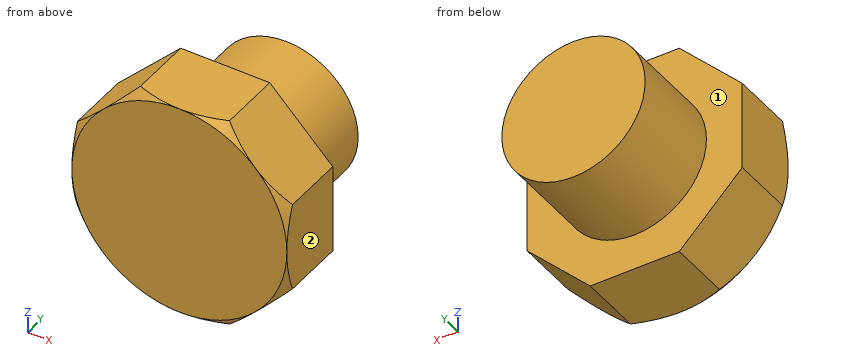
from build123d import *

# Parameters (mm, degrees)
SKETCH1_R           = 15
BOSS_EXTRUDE1_DEPTH = 20
BOSS_EXTRUDE2_DEPTH = 15
SKETCH3_OUTSIDE_W   = 101.526
SKETCH3_OUTSIDE_H   = 101.526
SKETCH3_OUTSIDE_R   = 22.5
CUT_EXTRUDE1_DEPTH  = 20
CUT_EXTRUDE1_DRAFT  = -45


with BuildPart() as part:
    # Sketch1 → Boss-Extrude1 (new body)
    with BuildSketch(Plane(origin=(0, 0, 0), x_dir=(1, 0, 0), z_dir=(0, 1, 0))):
        with Locations(Location((0, 0, 0), (0, 0, 270))):
            Circle(SKETCH1_R)
    extrude(amount=BOSS_EXTRUDE1_DEPTH)

    # Sketch2 → Boss-Extrude2 (add)
    with BuildSketch(Plane.XZ):
        Polygon((22.5, -9.319805153), (22.5, 9.319805153), (9.319805153, 22.5), (-9.319805153, 22.5), (-22.5, 9.319805153), (-22.5, -9.319805153), (-9.319805153, -22.5), (9.319805153, -22.5), align=None)
    extrude(amount=BOSS_EXTRUDE2_DEPTH)


with BuildPart() as cut_extrude1_tool:
    # Sketch3 outside → Cut-Extrude1 (with draft: the straight prism first)
    with BuildSketch(Plane(origin=(0, -15, 0), x_dir=(-1, 0, 0), z_dir=(0, -1, 0))):
        Rectangle(SKETCH3_OUTSIDE_W, SKETCH3_OUTSIDE_H)
        Circle(SKETCH3_OUTSIDE_R, mode=Mode.SUBTRACT)
    extrude(amount=-CUT_EXTRUDE1_DEPTH)
    # Cut-Extrude1: the draft: its side faces are tilted about the plane it starts from
    cut_extrude1_sides = [cut_extrude1_tool.faces().sort_by_distance(p)[0] for p in [
        (0, -5, 50.763),
        (-50.763, -5, 0),
        (0, -5, -50.763),
        (50.763, -5, 0),
        (22.5, -5, 0),
    ]]
    draft(cut_extrude1_sides, Plane(origin=(0, -15, 0), x_dir=(-1, 0, 0), z_dir=(0, -1, 0)), CUT_EXTRUDE1_DRAFT)


with BuildPart() as part_1:
    add(part.part)

    # Cut-Extrude1: cut by cut_extrude1_tool
    add(cut_extrude1_tool.part, mode=Mode.SUBTRACT)


solid = part_1.part
CAD build for the part. Positions are in the model's coordinates, mm. Face numbers are marked on the shaded views. A direction names the side the tool comes from. Give positions to 0.01 mm unless a question says otherwise; leave off trailing zeros. Loops run counter-clockwise (first coordinate to the right, second up) from the corner with the lowest first, then second, coordinate; pieces in that order, holes last. Notation, with made-up numbers: M -30,13.5 L 12,13.5 A27 ccw 12,29.5 Z; hole C 30.25,48.5 d1. An arc over 180 degrees is marked long. Answer in a Markdown table with one row per item. Add a question column.
Item 1: Tool access for the marked faces 1 and 2: list every direction of +Z, -Z, +X, -X, +Y, -Y with a clear straight run to the whole face (end or side of a thin tool).
Item 2: Probe probe 1 along Y at (x, z) = (10, 20); probe 2 along Z at (x, y) = (7.5, 10); probe 3 along X at (y, z) = (18, 11). List the from-to ranges inside material, lowest first.
Item 3: Band-saw the part on B-B on y = 12. Give the cut face in (x, z).
Item 4: Band-saw the part on A-A on y = -9.5. Give the cut face in (x, z), then the cut area to 3 significant figures.
Item 5: Drop flat-ended pins along their axis: P1, Ø8, axis at x = -10, y = 15, coming from the -Z side; P2, Ø1, axis at x = 10.5, y = 13, coming from the -Z side; P3, Ø3, axis at x = 12, y = 0, coming from the -Z side; P4, Ø6, axis at y = -1, z = -11.5, coming from the -X side. Give the stop position or say it passes through.
Reply:
| question | item | result |
|---|---|---|
| 1 | face 1 | +Y |
| 1 | face 2 | +Z, -Z, +X, +Y, -Y |
| 2 | probe 1 | y = -15 to 0 |
| 2 | probe 2 | z = -12.99 to 12.99 |
| 2 | probe 3 | x = -10.2 to 10.2 |
| 3 | outline | C 0,0 d30 |
| 4 | outline | M -22.5,-9.32 L -9.32,-22.5 L 9.32,-22.5 L 22.5,-9.32 L 22.5,9.32 L 9.32,22.5 L -9.32,22.5 L -22.5,9.32 Z |
| 4 | area | 1,680 mm^2 |
| 5 | P1 | stops at z = -13.75 |
| 5 | P2 | stops at z = -11.18 |
| 5 | P3 | stops at z = -21.32 |
| 5 | P4 | stops at x = -22.5 |
